from build123d import *

# Parameters (mm, degrees)
F1_R         = 27.5
F2_DEPTH     = 6.3
F3_W         = 9.4
F3_H         = 9.4
F4_DEPTH     = 10
F5_W         = 9.4
F5_H         = 3
F6_DEPTH     = 10
F7_R         = 2
F8_DEPTH     = 25
F9_R         = 4
F10_T1_DEPTH = 20
F11_R        = 4
F12_W        = 14
F12_H        = 3
F13_DEPTH    = 25
F14_W        = 14
F14_H        = 3
F15_DEPTH    = 25


# Not quite as in the source:
# - a fillet or chamfer that OpenCascade refuses, or shapes differently, is made with other operations: its cross-section is extruded or revolved along the edge and cut away or added


with BuildPart() as f2:
    # F1 (on offset) → F2 (new body)
    with BuildSketch(Plane.XY.offset(3.6)):
        Circle(F1_R)
    extrude(amount=F2_DEPTH)

    # F3 (on face) → F4 (join)
    with BuildSketch(Plane.XY.offset(9.9)):
        Rectangle(F3_W, F3_H)
    extrude(amount=F4_DEPTH)

    # F5 (on face) → F6 (join)
    with BuildSketch(Plane.XY.offset(19.9)):
        Rectangle(F5_W, F5_H)
    extrude(amount=F6_DEPTH)

    # F7 (on face) → F8 (cut)
    with BuildSketch(Plane.XZ.offset(1.5)):
        with Locations((0, 24.9)):
            Circle(F7_R)
    extrude(amount=-F8_DEPTH, mode=Mode.SUBTRACT)

    # F9
    f9_edges = [f2.edges().sort_by_distance(p)[0] for p in [
        (-4.7, 0, 29.9),
        (4.7, 0, 29.9),
    ]]
    fillet(f9_edges, radius=F9_R)

    # F10: fillet of radius 4 on 4 edges, made by hand

    # F10_s2 → F10_t1 (cut)
    with BuildSketch(Plane.XY.offset(9.9)):
        with BuildLine():
            ThreePointArc((-0.7, -4.7), (-3.5284271247, -3.5284271247), (-4.7, -0.7))
            Line((-4.7, -0.7), (-4.7, -4.7))
            Line((-4.7, -4.7), (-0.7, -4.7))
        make_face()
        with BuildLine():
            ThreePointArc((-0.7, 4.7), (-3.5284271247, 3.5284271247), (-4.7, 0.7))
            Line((-4.7, 0.7), (-4.7, 4.7))
            Line((-4.7, 4.7), (-0.7, 4.7))
        make_face()
        with BuildLine():
            ThreePointArc((4.7, -0.7), (3.5284271247, -3.5284271247), (0.7, -4.7))
            Line((0.7, -4.7), (4.7, -4.7))
            Line((4.7, -4.7), (4.7, -0.7))
        make_face()
        with BuildLine():
            ThreePointArc((4.7, 0.7), (3.5284271247, 3.5284271247), (0.7, 4.7))
            Line((0.7, 4.7), (4.7, 4.7))
            Line((4.7, 4.7), (4.7, 0.7))
        make_face()
    extrude(amount=F10_T1_DEPTH, mode=Mode.SUBTRACT)

    # F11
    f11_edges = [f2.edges().sort_by_distance(p)[0] for p in [
        (-3.528427, -3.528427, 9.9),
    ]]
    fillet(f11_edges, radius=F11_R)

    # F12 (on face) → F13 (cut)
    with BuildSketch(Plane(origin=(0, 4.7, 0), x_dir=(-1, 0, 0), z_dir=(0, 1, 0))):
        with Locations((-15.4635200504, 6.6790340934)):
            Rectangle(F12_W, F12_H)
    extrude(amount=F13_DEPTH, mode=Mode.SUBTRACT)

    # F14 (on face) → F15 (cut)
    with BuildSketch(Plane.XZ.offset(4.7)):
        with Locations((-15.1143019667, 6.7091025412)):
            Rectangle(F14_W, F14_H)
    extrude(amount=F15_DEPTH, mode=Mode.SUBTRACT)


solid = f2.part
Can you work these out from the model? Positions are in its coordinate system, mm. A direction names the side the tool comes from. Round coordinates to 2 decimals unless told otherwise and drop trailing zeros. Loops run counter-clockwise (first coordinate to the right, second up) from the corner with the lowest first, then second, coordinate; pieces in that order, holes last. Notation, with made-up numbers: (-12.75, -34.5) - (-5.75, -34.5) arc R24 ccw to (-5.75, -12.5) - close; hole circle Ø11 at (77.5, 39.5). An arc over 180 degrees is marked (long way). Answer in a Markdown table with one row per item. Add a question column.
Q1. I want a section at A-A on x = 0. List the corners of the cut face in (y, z) for me.
Q2. I want a section at B-B on z = 24.9. List the corners of the cut face in (x, y) for me.
Q3. Which directions (+Z, -Z, +X, -X, +Y, -Y) give clear straight access to the entire face, cutting with the end or side of a thin tool? Please do faces 1 (the flat face through (-8.114, -15, 7)), 2 (the cylindrical face through (-3.95, -3.03, 17.37)), 3 (the cylindrical face through (4, 2.96, 17.37)).
Q4. I need wall thicknesses on L1, parallel to Z at x = -21, y = -11; L2, parallel to Z at x = 0, y = 0; L3, parallel to Z at x = -3, y = -25. Which ranges of each line are inside material? Lowest first, please.
Q5. For pin 1 Ø2 at (x, y) = (7.5, -16.5) entering from +Z; pin 2 Ø4.5 at (x, z) = (2, 23.5) entering from +Y; pin 3 Ø1 at (x, y) = (-0.5, 4) entering from +Z, each with a flat end and sliding along its axis, tell me the tip position at first contact or that it passes through.
Q6. I want a section at D-D on z = 6.5. List the corners of the cut face in (x, y) for me, and give its area (3 significant figures).
Q7. We'd pull the mould along X, two halves only. Please class faces 4 (the cylindrical face through (5.903, -0.01, 11.041)), 5 (the cylindrical face through (0.01, 5.903, 11.041)), 6 (the cylindrical face through (-0.26, -0.021, 26.883)): pulls with the +X half, pulls with the -X half, needs draft (parallel to the pull), parting line crosses it, or undercut.
Q8. I want a section at C-C on y = 0. List the corners of the cut face in (x, z) for me, and give its area (3 significant figures).
A:
| question | item | result |
|---|---|---|
| 1 | outline | (-27.5, 3.6) - (27.5, 3.6) - (27.5, 9.9) - (8.7, 9.9) arc R4 cw to (4.7, 13.9) - (4.7, 19.9) - (1.5, 19.9) - (1.5, 22.9) - (-1.5, 22.9) - (-1.5, 19.9) - (-4.7, 19.9) - (-4.7, 13.9) arc R4 cw to (-8.7, 9.9) - (-27.5, 9.9) - close; (-1.5, 26.9) - (1.5, 26.9) - (1.5, 29.9) - (-1.5, 29.9) - close |
| 2 | outline | (-4.7, -0.7) arc R4 ccw to (-4.62, -1.5) - (-2, -1.5) - (-2, 1.5) - (-4.62, 1.5) arc R4 ccw to (-4.7, 0.7) - close; (2, -1.5) - (4.62, -1.5) arc R4 ccw to (4.7, -0.7) - (4.7, 0.7) arc R4 ccw to (4.62, 1.5) - (2, 1.5) - close |
| 3 | face 1 | -Y |
| 3 | face 2 | +Z, -X, -Y |
| 3 | face 3 | +Z, +X, +Y |
| 4 | L1 | 3.6 to 5.21, 8.21 to 9.9 |
| 4 | L2 | 3.6 to 22.9, 26.9 to 29.9 |
| 4 | L3 | 3.6 to 9.9 |
| 5 | pin 1 | z = 9.9 |
| 5 | pin 2 | y = 1.5 |
| 5 | pin 3 | z = 19.9 |
| 6 | outline | (-22.11, -16.35) - (-22.11, -4.7) - (-8.11, -4.7) - (-8.11, -26.28) arc R27.5 ccw to (22.46, 15.86) - (22.46, 4.7) - (8.46, 4.7) - (8.46, 26.17) arc R27.5 ccw to start |
| 6 | area | 1,880 mm^2 |
| 7 | face 4 | pulls with the +X half |
| 7 | face 5 | needs draft |
| 7 | face 6 | undercut |
| 8 | outline | (-27.5, 3.6) - (27.5, 3.6) - (27.5, 9.9) - (8.7, 9.9) arc R4 cw to (4.7, 13.9) - (4.7, 25.9) arc R4 ccw to (0.7, 29.9) - (-0.7, 29.9) arc R4 ccw to (-4.7, 25.9) - (-4.7, 13.9) arc R4 cw to (-8.7, 9.9) - (-27.5, 9.9) - close; hole circle Ø4 at (0, 24.9) |
| 8 | area | 522 mm^2 |
